Here's how the part is built. I have some questions about the finished solid (model axes, mm). A direction names the side the tool comes from. Give positions to 0.01 mm unless a question says otherwise; leave off trailing zeros. Write each loop counter-clockwise with the first axis right and the second up, starting at its lowest first coordinate (ties: lowest second). Pieces come first, ordered by that corner, then holes. Notation, with made-up numbers: (72.25, -30.75) - (82.25, -30.75) arc R29 ccw to (82.25, 1.25) - close; hole circle Ø1 at (55.5, 31). An arc over 180 degrees is marked (long way). One line per item, written item: value. Start each with the question number.
1) I'm going to push flat-ended pins straight in: P1, Ø11.5, axis at x = 1.5, y = 19.5, coming from the +Z side; P2, Ø4.5, axis at x = -19.1, y = 29.64, coming from the +Z side; P3, Ø5, axis at x = -21, y = 31, coming from the +Z side; P4, Ø5.5, axis at x = -33.35, y = -18.67, coming from the +Z side. Where does each tip first touch, or does it pass through?
2) Imagine slicing it at A-A on x = -9. Write out the boundary of the cut face in (y, z), plus the area to 3 significant figures.
3) We'd pull the mould along Y, two halves only. Please class faces 5 (the cylindrical face through (-16.37, 33.92, -35.94)), 6 (the cylindrical face through (40.551, -0.764, 5.596)), 7 (the cylindrical face through (-40.511, 22.307, -35.014)): +Y half, -Y half, draft (parallel to the pull), parting line (faces both ways), or undercut.
4) On a 3-axis mill with a long thin cutter (end or side, diameter ignored), from which of +Z, -Z, +X, -X, +Y, -Y can I reach the whole of each face in a straight line? I mean faces 1 (the cylindrical face through (35.13, -17.04, -2.28)), 2 (the flat face through (1, 22, -34.29)), 3 (the cylindrical face through (29.32, -21.76, 42.8)), 4 (the cylindrical face through (-40.511, -0.724, 5.596)). Say none if no direction works.
5) Imagine slicing it at D-D on z = -23.5. Write out the boundary of the cut face in (x, y) (3 decimals).
6) Please list where these lines run through material, in increasing order: L1, parallel to Y at x = -33, z = 14.5; L2, parallel to Y at x = 36, z = -0.5; L3, parallel to Z at x = -11, y = 6.5. Write a range as [from, to].
7) Imagine slicing it at C-C on y = 37. Write out the boundary of the cut face in (x, z) (3 decimals).
8) Imagine slicing it at B-B on x = -18. Write out the boundary of the cut face in (y, z).
from build123d import *

# Parameters (mm, degrees)
F0_W           = 82.55
F0_H           = 88.9
F1_DEPTH       = 44.069
F2_W           = 82.55
F2_H           = 10.16
F3_DEPTH       = 44.069
F5_D           = 4.826
F5_CBORE_D     = 10.16
F5_CBORE_DEPTH = 3.3528
F6_R           = 2.54
F8_D           = 4.826
F8_CBORE_D     = 10.16
F8_CBORE_DEPTH = 3.3528


# Not quite as in the source:
# - a feature names something its author has since deleted; it is built from what else it names


with BuildPart() as f1:
    # F0 (on Front) → F1 (new body)
    with BuildSketch(Plane.XZ):
        Rectangle(F0_W, F0_H)
    extrude(amount=F1_DEPTH)

    # F2 (on face) → F3 (join)
    with BuildSketch(Plane(origin=(0, 0, 0), x_dir=(-1, 0, 0), z_dir=(0, 1, 0))):
        with Locations((0, -39.37)):
            Rectangle(F2_W, F2_H)
    extrude(amount=F3_DEPTH)

    # F5 (through all)
    with Locations(Plane.XY.offset(44.45)):
        with Locations((-33.3502, -18.669), (33.3502, -18.669)):
            CounterBoreHole(F5_D / 2, F5_CBORE_D / 2, F5_CBORE_DEPTH)

    # F6
    f6_edges = [f1.edges().sort_by_distance(p)[0] for p in [
        (-41.275, -22.0345, 44.45),
        (41.275, -22.0345, 44.45),
        (0, -44.069, 44.45),
        (0, 0, 44.45),
        (41.275, -44.069, 0),
        (41.275, 0, 5.08),
        (-41.275, -44.069, 0),
        (-41.275, 0, 5.08),
        (-41.275, 22.0345, -34.29),
        (0, 44.069, -34.29),
        (41.275, 22.0345, -34.29),
        (0, 0, -34.29),
        (41.275, 44.069, -39.37),
        (-41.275, 44.069, -39.37),
    ]]
    fillet(f6_edges, radius=F6_R)

    # F8 (through all)
    with Locations(Plane.XY.offset(-34.29)):
        with Locations((-19.1008, 29.6364016831), (19.0881, 29.6364016831)):
            CounterBoreHole(F8_D / 2, F8_CBORE_D / 2, F8_CBORE_DEPTH)


solid = f1.part
Numbers:
1. P1: z = -34.29
1. P2: through
1. P3: z = -37.64
1. P4: z = 41.1
2. outline: (-44.07, -44.45) - (44.07, -44.45) - (44.07, -36.83) arc R2.54 ccw to (41.53, -34.29) - (2.54, -34.29) arc R2.54 cw to (0, -31.75) - (0, 41.91) arc R2.54 ccw to (-2.54, 44.45) - (-41.53, 44.45) arc R2.54 ccw to (-44.07, 41.91) - close
2. area: 4,360 mm^2
3. face 5: undercut
3. face 6: +Y half
3. face 7: draft
4. face 1: +Z, -Z
4. face 2: +Z, +X, -X, +Y
4. face 3: +Z
4. face 4: +Z, -X, +Y
5. outline: (-41.275, -41.529) arc R2.54 ccw to (-38.735, -44.069) - (38.735, -44.069) arc R2.54 ccw to (41.275, -41.529) - (41.275, -2.54) arc R2.54 ccw to (38.735, 0) - (-38.735, 0) arc R2.54 ccw to (-41.275, -2.54) - close; hole circle Ø4.826 at (-33.35, -18.669); hole circle Ø4.826 at (33.35, -18.669)
6. L1: [-44.07, -21.06], [-16.28, 0]
6. L2: [-44.07, 0]
6. L3: [-44.45, -34.29]
7. outline: (-41.275, -44.45) - (41.275, -44.45) - (41.275, -36.83) arc R2.54 ccw to (38.735, -34.29) - (-38.735, -34.29) arc R2.54 ccw to (-41.275, -36.83) - close
8. outline: (-44.07, -44.45) - (27.49, -44.45) - (27.49, -37.64) - (24.68, -37.64) - (24.68, -34.29) - (2.54, -34.29) arc R2.54 cw to (0, -31.75) - (0, 41.91) arc R2.54 ccw to (-2.54, 44.45) - (-41.53, 44.45) arc R2.54 ccw to (-44.07, 41.91) - close; (31.78, -44.45) - (44.07, -44.45) - (44.07, -36.83) arc R2.54 ccw to (41.53, -34.29) - (34.6, -34.29) - (34.6, -37.64) - (31.78, -37.64) - close
